from build123d import *

# Parameters (mm, degrees)
SKETCH1_R           = 14
BOSS_EXTRUDE1_DEPTH = 3
SKETCH2_OUTSIDE_W   = 194.236
SKETCH2_OUTSIDE_H   = 194.236
SKETCH2_OUTSIDE_W_2 = 89.848932168
SKETCH2_OUTSIDE_H_2 = 89.848932168
CUT_EXTRUDE1_DEPTH  = 3
BOSS_EXTRUDE2_DEPTH = 3


with BuildPart() as part:
    # Sketch1 → Boss-Extrude1 (new body)
    with BuildSketch(Plane.XY):
        Polygon((0.667250758, 74.924466084), (-74.924466084, -0.667250758), (-0.667250758, -74.924466084), (74.924466084, 0.667250758), align=None)
        Circle(SKETCH1_R, mode=Mode.SUBTRACT)
        with BuildLine():
            Line((36.187095947, -23.927983755), (23.927983755, -36.187095947))
            ThreePointArc((23.927983755, -36.187095947), (15.242424375, -37.934763642), (10.271443313, -30.601099389))
            Line((10.271443313, -30.601099389), (10.161887104, -18.232430989))
            ThreePointArc((10.161887104, -18.232430989), (12.504719048, -12.504719048), (18.232430989, -10.161887104))
            Line((18.232430989, -10.161887104), (30.601099389, -10.271443313))
            ThreePointArc((30.601099389, -10.271443313), (37.934763642, -15.242424375), (36.187095947, -23.927983755))
        make_face(mode=Mode.SUBTRACT)
        with BuildLine():
            Line((-23.927983755, 36.187095947), (-36.187095947, 23.927983755))
            ThreePointArc((-36.187095947, 23.927983755), (-37.934763642, 15.242424375), (-30.601099389, 10.271443313))
            Line((-30.601099389, 10.271443313), (-18.232430989, 10.161887104))
            ThreePointArc((-18.232430989, 10.161887104), (-12.504719048, 12.504719048), (-10.161887104, 18.232430989))
            Line((-10.161887104, 18.232430989), (-10.271443313, 30.601099389))
            ThreePointArc((-10.271443313, 30.601099389), (-15.242424375, 37.934763642), (-23.927983755, 36.187095947))
        make_face(mode=Mode.SUBTRACT)
        with BuildLine():
            Line((-38.079203745, -23.370377474), (-23.370377474, -38.079203745))
            ThreePointArc((-23.370377474, -38.079203745), (-14.619353482, -39.79975511), (-9.713837032, -32.351491804))
            Line((-9.713837032, -32.351491804), (-9.842977457, -17.771805959))
            ThreePointArc((-9.842977457, -17.771805959), (-12.185809401, -12.185809401), (-17.771805959, -9.842977457))
            Line((-17.771805959, -9.842977457), (-32.351491804, -9.713837032))
            ThreePointArc((-32.351491804, -9.713837032), (-39.79975511, -14.619353482), (-38.079203745, -23.370377474))
        make_face(mode=Mode.SUBTRACT)
        with BuildLine():
            Line((9.713837032, 32.351491804), (9.842977457, 17.771805959))
            ThreePointArc((9.842977457, 17.771805959), (12.185809401, 12.185809401), (17.771805959, 9.842977457))
            Line((17.771805959, 9.842977457), (32.351491804, 9.713837032))
            ThreePointArc((32.351491804, 9.713837032), (39.79975511, 14.619353482), (38.079203745, 23.370377474))
            Line((38.079203745, 23.370377474), (23.370377474, 38.079203745))
            ThreePointArc((23.370377474, 38.079203745), (14.619353482, 39.79975511), (9.713837032, 32.351491804))
        make_face(mode=Mode.SUBTRACT)
    extrude(amount=BOSS_EXTRUDE1_DEPTH)

    # Sketch2 outside → Cut-Extrude1 (cut)
    with BuildSketch(Plane.XY.offset(3)):
        Rectangle(SKETCH2_OUTSIDE_W, SKETCH2_OUTSIDE_H)
        Rectangle(SKETCH2_OUTSIDE_W_2, SKETCH2_OUTSIDE_H_2, mode=Mode.SUBTRACT)
    extrude(amount=-CUT_EXTRUDE1_DEPTH, mode=Mode.SUBTRACT)

    # Sketch3 → Boss-Extrude2 (add)
    with BuildSketch(Plane.XY.offset(3)):
        with BuildLine():
            Line((-80, -100), (-67.193751525, -100))
            Line((-67.193751525, -100), (-26.135764012, -48.677515609))
            ThreePointArc((-26.135764012, -48.677515609), (-22.658963222, -45.911433721), (-18.327075918, -44.924466084))
            Line((-18.327075918, -44.924466084), (-30.667250758, -44.924466084))
            Line((-30.667250758, -44.924466084), (-47.039809367, -28.551907475))
            ThreePointArc((-47.039809367, -28.551907475), (-44.126179551, -35.06997143), (-46.302189085, -41.869925762))
            Line((-46.302189085, -41.869925762), (-80, -83.992189406))
            Line((-80, -83.992189406), (-80, -100))
        make_face()
        with BuildLine():
            Line((29.332749242, -44.924466084), (18.327075918, -44.924466084))
            ThreePointArc((18.327075918, -44.924466084), (22.658963222, -45.911433721), (26.135764012, -48.677515609))
            Line((26.135764012, -48.677515609), (67.193751525, -100))
            Line((67.193751525, -100), (80, -100))
            Line((80, -100), (80, -83.992189406))
            Line((80, -83.992189406), (45.7090773, -41.128536031))
            ThreePointArc((45.7090773, -41.128536031), (43.533067766, -34.328581698), (46.446697582, -27.810517744))
            Line((46.446697582, -27.810517744), (29.332749242, -44.924466084))
        make_face()
        with BuildLine():
            Line((-46.446697582, 27.810517744), (-29.332749242, 44.924466084))
            Line((-29.332749242, 44.924466084), (-18.327075918, 44.924466084))
            ThreePointArc((-18.327075918, 44.924466084), (-22.658963222, 45.911433721), (-26.135764012, 48.677515609))
            Line((-26.135764012, 48.677515609), (-67.193751525, 100))
            Line((-67.193751525, 100), (-80, 100))
            Line((-80, 100), (-80, 83.992189406))
            Line((-80, 83.992189406), (-45.7090773, 41.128536031))
            ThreePointArc((-45.7090773, 41.128536031), (-43.533067766, 34.328581698), (-46.446697582, 27.810517744))
        make_face()
        with BuildLine():
            Line((30.667250758, 44.924466084), (47.039809367, 28.551907475))
            ThreePointArc((47.039809367, 28.551907475), (44.126179551, 35.06997143), (46.302189085, 41.869925762))
            Line((46.302189085, 41.869925762), (80, 83.992189406))
            Line((80, 83.992189406), (80, 100))
            Line((80, 100), (67.193751525, 100))
            Line((67.193751525, 100), (26.135764012, 48.677515609))
            ThreePointArc((26.135764012, 48.677515609), (22.658963222, 45.911433721), (18.327075918, 44.924466084))
            Line((18.327075918, 44.924466084), (30.667250758, 44.924466084))
        make_face()
    extrude(amount=-BOSS_EXTRUDE2_DEPTH)


solid = part.part
The model under review builds one solid part; all positions refer to its coordinate system, in mm. A direction names the side the tool comes from. Round coordinates to 2 decimals unless told otherwise and drop trailing zeros. Loops run counter-clockwise (first coordinate to the right, second up) from the corner with the lowest first, then second, coordinate; pieces in that order, holes last. Notation, with made-up numbers: (-28.75, 65) -> (7.25, 65) arc R20 cw to (7.25, 76) -> close; hole circle Ø11 at (2, -23.5). An arc over 180 degrees is marked (long way). Return JSON: item names as keys, results as strings.
(1) The part is to be moulded in two halves that separate along Y. For faces 1 (the cylindrical face through (37.884, -15.121, 1.479)), 2 (the flat face through (-46.38, 73.98, 1.52)), 3 (the flat face through (46.38, -73.98, 1.52)), say which applies: released by +Y, released by -Y, zero draft, split by the parting line, or undercut.
Solved:
{"face 1": "undercut", "face 2": "released by +Y", "face 3": "released by -Y"}
(2) For line 1 (X direction, y = -32, z = 1.2); line 2 (Y direction, x = 0, z = 2.25); line 3 (X direction, y = 22, z = 1.6), list the stretches that pass through material, from the lowest coordinate up.
Solved:
{"line 1": "-44.79 to -29.45, -9.72 to 10.41, 28.12 to 43.94", "line 2": "-44.92 to -14, 14 to 44.92", "line 3": "-44.92 to -37.61, -10.2 to 9.81, 39.18 to 44.92"}
(3) Add section A-A on x = 0. Write out the cut boundary in (y, z), plus the area to 3 significant figures.
Solved:
{"outline": "(-44.92, 0) -> (-14, 0) -> (-14, 3) -> (-44.92, 3) -> close; (14, 0) -> (44.92, 0) -> (44.92, 3) -> (14, 3) -> close", "area": "186 mm2"}
(4) Add section C-C on z = 1.1. State how many separate pieces and enclosed holes the cut face has, plus the area to 3 significant figures.
Solved:
{"separate pieces": "1", "enclosed holes": "5", "area": "10,100 mm2"}
(5) For pin 1 (1.5 mm diameter, centred on y = -45.5, z = 1, fed in from +X); pin 2 (1 mm diameter, centred on y = -36, z = 2.5, fed in from -X); pin 3 (22.5 mm diameter, centred on x = 0, y = 0, fed in from +Z); pin 4 (0.9 mm diameter, centred on y = 13, z = 2, fed in from +X), all flat-tipped, find the tip position at first contact; note any pin that passes through.
Solved:
{"pin 1": "x = 49.81", "pin 2": "x = -44.15", "pin 3": "through", "pin 4": "x = 44.92"}
(6) For faces 4 (the flat face through (-46.952, -74.698, 1.521)), 5 (the flat face through (-18, 0, 0)), 6 (the cylindrical face through (-39.75, -14.5, 1.48)), 7 (the flat face through (62.92, 62.64, 1.52)), 8 (the flat face through (-63.095, 62.86, 1.521)), list the 3-axis set-ups (+Z, -Z, +X, -X, +Y, -Y) from which the entire face can be reached by the end or side of a thin tool; tool diameter is ignored.
Solved:
{"face 4": "+Z, -Z, -Y", "face 5": "-Z, +X, -X, +Y, -Y", "face 6": "+Z, -Z", "face 7": "+Z, -Z, +X", "face 8": "+Z, -Z, -X"}
